Read the model definition and answer for the solid it produces. Units are mm, in the model's axes. Coordinates: 2 decimals unless noted, no trailing zeros.
from build123d import *

# Parameters (mm, degrees)
SKETCH1_R           = 2
SKETCH1_W           = 12
SKETCH1_H           = 4.5
SKETCH1_W_2         = 61.5
SKETCH1_H_2         = 61.5
SKETCH1_W_3         = 30
SKETCH1_H_3         = 20
SKETCH1_W_4         = 15
SKETCH1_H_4         = 5
BOSS_EXTRUDE1_DEPTH = 5


with BuildPart() as part:
    # Sketch1 → Boss-Extrude1 (new body)
    with BuildSketch(Plane.XY):
        Polygon((148, -50), (168, -50), (168, -30), (163, -30), (163, 30), (168, 30), (168, 50), (148, 50), (148, 55), (98, 55), (98, 50), (50, 50), (50, 55), (-50, 55), (-50, 50), (-98, 50), (-98, 55), (-148, 55), (-148, 50), (-168, 50), (-168, 30), (-163, 30), (-163, -30), (-168, -30), (-168, -50), (-148, -50), (-148, -55), (-98, -55), (-98, -50), (-50, -50), (-50, -55), (50, -55), (50, -50), (98, -50), (98, -55), (148, -55), align=None)
        with Locations((-20, -35.75)):
            Circle(SKETCH1_R, mode=Mode.SUBTRACT)
        with Locations((-65, -22.25)):
            Rectangle(SKETCH1_W, SKETCH1_H, mode=Mode.SUBTRACT)
        with Locations((51.5, -35.75)):
            Circle(SKETCH1_R, mode=Mode.SUBTRACT)
        with Locations((71.5, -35.75)):
            Circle(SKETCH1_R, mode=Mode.SUBTRACT)
        with Locations((143, -35.75)):
            Circle(SKETCH1_R, mode=Mode.SUBTRACT)
        with Locations((15.75, 0)):
            Rectangle(SKETCH1_W_2, SKETCH1_H_2, mode=Mode.SUBTRACT)
        with Locations((-65, 0)):
            Rectangle(SKETCH1_W_3, SKETCH1_H_3, mode=Mode.SUBTRACT)
        with Locations((-65, 22.5)):
            Rectangle(SKETCH1_W_4, SKETCH1_H_4, mode=Mode.SUBTRACT)
        with Locations((-20, 35.75)):
            Circle(SKETCH1_R, mode=Mode.SUBTRACT)
        with Locations((107.25, 0)):
            Rectangle(SKETCH1_W_2, SKETCH1_H_2, mode=Mode.SUBTRACT)
        with Locations((51.5, 35.75)):
            Circle(SKETCH1_R, mode=Mode.SUBTRACT)
        with Locations((71.5, 35.75)):
            Circle(SKETCH1_R, mode=Mode.SUBTRACT)
        with Locations((143, 35.75)):
            Circle(SKETCH1_R, mode=Mode.SUBTRACT)
    extrude(amount=BOSS_EXTRUDE1_DEPTH)


solid = part.part
Item 1: The part is cut by section A-A (z = 1.3). State how many separate pieces and enclosed holes the cut face has, and give its area (3 significant figures).
Item 2: Find the intervals of material crossed by probe 1 along X at (y, z) = (14.5, 4.25); probe 2 along Y at (x, z) = (-66.5, 4.8); probe 3 along X at (y, z) = (-4.5, 3.35), in increasing order.
Item 3: Given pin 1 (1.5 mm diameter, centred on x = -54, z = 3.5, fed in from +Y); pin 2 (1 mm diameter, centred on x = -130.5, y = 35.5, fed in from -Z); pin 3 (2.5 mm diameter, centred on y = -53.5, z = 3, fed in from -X); pin 4 (2 mm diameter, centred on y = 14, z = 4.5, fed in from +X), each flat-ended and moving along its own axis, determine where each tip first touches the part or whether it passes through.
Answer:
1. separate pieces: 1
1. enclosed holes: 13
1. area: 26,600 mm2
2. probe 1: x = -163 to -15, 46.5 to 76.5, 138 to 163
2. probe 2: y = -50 to -24.5, -20 to -10, 10 to 20, 25 to 50
2. probe 3: x = -163 to -80, -50 to -15, 46.5 to 76.5, 138 to 163
3. pin 1: stops at y = 50
3. pin 2: stops at z = 0
3. pin 3: stops at x = -148
3. pin 4: stops at x = 163
